The model under review builds one solid part; all positions refer to its coordinate system, in mm. Face numbers are marked on the shaded views. Coordinates: 2 decimals unless noted, no trailing zeros. Loops run counter-clockwise (first coordinate to the right, second up) from the corner with the lowest first, then second, coordinate; pieces in that order, holes last. Notation, with made-up numbers: M -28.5,-27.5 L 12.5,-27.5 A23 cw 12.5,-8.5 Z; hole C 18.5,73.25 d6. An arc over 180 degrees is marked long. Return JSON: item names as keys, results as strings.
```python
from build123d import *

# Parameters (mm, degrees)
SKETCH1_W           = 50
SKETCH1_H           = 50
BOSS_EXTRUDE1_DEPTH = 4
SKETCH2_R           = 8.2
SKETCH2_R_2         = 1
CUT_EXTRUDE1_DEPTH  = 10
SKETCH3_R           = 1
CUT_EXTRUDE2_DEPTH  = 4
FILLET1_R           = 10


with BuildPart() as part:
    # Sketch1 → Boss-Extrude1 (new body)
    with BuildSketch(Plane.XY):
        Rectangle(SKETCH1_W, SKETCH1_H)
    extrude(amount=BOSS_EXTRUDE1_DEPTH)

    # Sketch2 → Cut-Extrude1 (cut)
    with BuildSketch(Plane.XY.offset(4)):
        Circle(SKETCH2_R)
        with Locations((-8, 7.5)):
            Circle(SKETCH2_R_2)
        with Locations((8, 7.5)):
            Circle(SKETCH2_R_2)
        with Locations((-8, -22.5)):
            Circle(SKETCH2_R_2)
        with Locations((8, -22.5)):
            Circle(SKETCH2_R_2)
    extrude(amount=-CUT_EXTRUDE1_DEPTH, mode=Mode.SUBTRACT)

    # Sketch3 → Cut-Extrude2 (cut)
    with BuildSketch(Plane.XY.offset(4)):
        with Locations((-17.67766953, 17.67766953)):
            Circle(SKETCH3_R)
        with Locations((17.67766953, 17.67766953)):
            Circle(SKETCH3_R)
        with Locations((17.67766953, -17.67766953)):
            Circle(SKETCH3_R)
        with Locations((-17.67766953, -17.67766953)):
            Circle(SKETCH3_R)
    extrude(amount=-CUT_EXTRUDE2_DEPTH, mode=Mode.SUBTRACT)

    # Fillet1
    fillet1_edges = [part.edges().sort_by_distance(p)[0] for p in [
        (25, -25, 2),
        (-25, -25, 2),
        (-25, 25, 2),
        (25, 25, 2),
    ]]
    fillet(fillet1_edges, radius=FILLET1_R)


solid = part.part
```
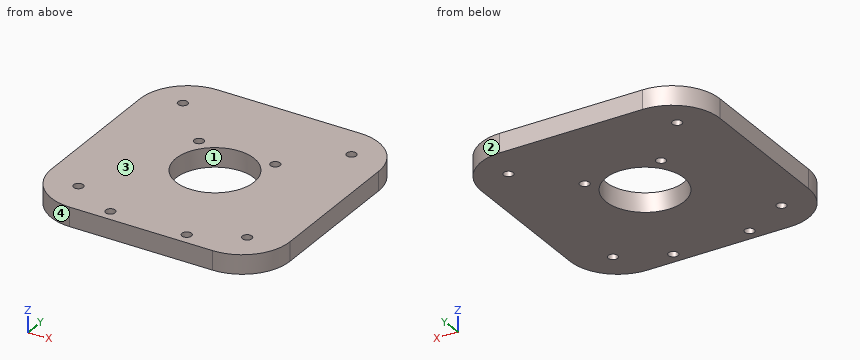
1. Add section C-C on z = 2.4. State how many separate pieces and enclosed holes the cut face has, plus the area to 3 significant figures.
Check values:
{"separate pieces": "1", "enclosed holes": "9", "area": "2,180 mm²"}
2. Add section D-D on y = -22.5. Give the boundary of the cut face in (x, z), plus the area to 3 significant figures.
Check values:
{"outline": "M -21.61,0 L -9,0 L -9,4 L -21.61,4 Z; M -7,0 L 7,0 L 7,4 L -7,4 Z; M 9,0 L 21.61,0 L 21.61,4 L 9,4 Z", "area": "157 mm²"}
3. Add section B-B on y = 3.5. Give the boundary of the cut face in (x, z), plus the area to 3 significant figures.
Check values:
{"outline": "M -25,0 L -7.42,0 L -7.42,4 L -25,4 Z; M 7.42,0 L 25,0 L 25,4 L 7.42,4 Z", "area": "141 mm²"}
4. Add section A-A on x = 0. Give the boundary of the cut face in (y, z).
Check values:
{"outline": "M -25,0 L -8.2,0 L -8.2,4 L -25,4 Z; M 8.2,0 L 25,0 L 25,4 L 8.2,4 Z"}
5. The part is to be moulded in two halves that separate along X. For the marked faces 1, 2, 3 and 4, say which applies: released by +X, released by -X, zero draft, split by the parting line, or undercut.
Check values:
{"face 1": "undercut", "face 2": "released by +X", "face 3": "zero draft", "face 4": "released by -X"}
6. To check wall thickness, follow line 1 (X direction, y = -17.5, z = 2.05); line 2 (X direction, y = -1, z = 1.45); line 3 (X direction, y = -17, z = 1.1). State the ranges of each line that lie inside material, in increasing order.
Check values:
{"line 1": "-24.68 to -18.66, -16.69 to 16.69, 18.66 to 24.68", "line 2": "-25 to -8.14, 8.14 to 25", "line 3": "-24.8 to -18.41, -16.94 to 16.94, 18.41 to 24.8"}
